Input: part model. Units: mm. Frame: model coordinates. Coordinates: 2 decimals unless noted, no trailing zeros. Write each loop counter-clockwise with the first axis right and the second up, starting at its lowest first coordinate (ties: lowest second). Pieces come first, ordered by that corner, then holes.
1) Section query D-D (x = 10). Output: boundary loops of the cut face in (y, z).
2) Section query C-C (x = 8). Output: boundary loops of the cut face in (y, z).
3) Section query A-A (z = 0). Output: boundary loops of the cut face in (x, y).
4) Line query: L1, parallel to Y at x = 4.75, z = -0.95; L2, parallel to Y at x = 9, z = 1.25; L3, parallel to X at y = -0.05, z = 1.6. Output: solid intervals per line, ascending.
5) Pin query (flat end, axial travel): pin 1 Ø2 at (x, z) = (7, -0.5) entering from -Y. Return the tip coordinate at first contact, or that it passes through.
from build123d import *

# Parameters (mm, degrees)
SKETCH1_W     = 11
SKETCH1_H     = 2
CHAMFER1_SIZE = 1
FILLET1_R     = 2


with BuildPart() as part:
    # Sketch1 → Revolve1 (revolve)
    with BuildSketch(Plane.XY):
        with Locations((5.5, 1)):
            Rectangle(SKETCH1_W, SKETCH1_H)
    revolve(axis=Axis((-4.801500481, 0, 0), (1, 0, 0)))

    # Chamfer1
    chamfer1_edges = [part.edges().sort_by_distance(p)[0] for p in [
        (0, -2, 0),
    ]]
    chamfer(chamfer1_edges, length=CHAMFER1_SIZE)

    # Fillet1
    fillet1_edges = [part.edges().sort_by_distance(p)[0] for p in [
        (11, -2, 0),
    ]]
    fillet(fillet1_edges, radius=FILLET1_R)


solid = part.part
Answer:
1. outline: circle Ø3.46 at (0, 0)
2. outline: circle Ø4 at (0, 0)
3. outline: (0, -1) - (1, -2) - (9, -2) arc R2 ccw to (9, 2) - (1, 2) - (0, 1) - close
4. L1: y = -1.76 to 1.76
4. L2: y = -1.56 to 1.56
4. L3: x = 0.6 to 10.2
5. pin 1: stops at y = -2
